Geometry: final body of the model. Coordinates: model frame, mm. A direction names the side the tool comes from. Round coordinates to 2 decimals unless told otherwise and drop trailing zeros. Loops run counter-clockwise (first coordinate to the right, second up) from the corner with the lowest first, then second, coordinate; pieces in that order, holes last. Notation, with made-up numbers: (50, 67.25) -> (71, 67.25) arc R30 cw to (71, 104.25) -> close; hole circle Ø4 at (72, -36.5). An arc over 180 degrees is marked (long way). Answer in a Markdown table with one row per item.
```python
from build123d import *

# Parameters (mm, degrees)
F0_W     = 2
F0_H     = 2.4
F1_DEPTH = 10
F2_DEPTH = 10


with BuildPart() as f1:
    # F0 (on Top) → F1 (new body)
    with BuildSketch(Plane.XY):
        with Locations((-8.5, 4.8)):
            Rectangle(F0_W, F0_H)
        Polygon((-11.5, 0), (-9.5, 0), (-9.5, 3.6), (-9.5, 6), (-11.5, 6), align=None)
        Polygon((9.5, 0), (0, 0), (0, -1.5), (11.5, -1.5), (11.5, 0), align=None)
        with Locations((8.5, 4.8)):
            Rectangle(F0_W, F0_H)
        Polygon((0, -1.5), (0, 0), (-9.5, 0), (-11.5, 0), (-11.5, -1.5), align=None)
        Polygon((9.5, 3.6), (9.5, 0), (11.5, 0), (11.5, 6), (9.5, 6), align=None)
    extrude(amount=F1_DEPTH)

    # F0 (on Top) → F2 (join)
    with BuildSketch(Plane.XY):
        Polygon((-11.5, -1.5), (-11.5, 0), (-11.5, 6), (-19, 6), (-16, -1.5), align=None)
        with BuildLine():
            Line((-31, 6), (-28, 6))
            Line((-28, 6), (-28, 28.5))
            Line((-28, 28.5), (-28, 53.5))
            ThreePointArc((-28, 53.5), (-33, 58.5), (-38, 53.5))
            Line((-38, 53.5), (-38, 23.5))
            Line((-38, 23.5), (-31, 6))
        make_face()
        Polygon((11.5, 0), (11.5, -1.5), (16, -1.5), (19, 6), (11.5, 6), align=None)
        with BuildLine():
            Line((28, 6), (31, 6))
            Line((31, 6), (38, 23.5))
            Line((38, 23.5), (38, 53.5))
            ThreePointArc((38, 53.5), (33, 58.5), (28, 53.5))
            Line((28, 53.5), (28, 28.5))
            Line((28, 28.5), (28, 6))
        make_face()
        Polygon((-28, 6), (-19, 6), (-28, 28.5), align=None)
        Polygon((-28, -1.5), (-16, -1.5), (-19, 6), (-28, 6), (-31, 6), align=None)
        Polygon((19, 6), (16, -1.5), (28, -1.5), (31, 6), (28, 6), align=None)
        Polygon((28, 28.5), (19, 6), (28, 6), align=None)
        Polygon((11.5, -1.5), (0, -1.5), (-11.5, -1.5), (-16, -1.5), (-28, -1.5), (-26.5144372946, -5.2139067635), (26.5144372946, -5.2139067635), (28, -1.5), (16, -1.5), align=None)
    extrude(amount=F2_DEPTH)


solid = f1.part
```
Item 1: Section query C-C, the plane x = 22.5. Output: boundary loops of the cut face in (y, z), and give its area (3 significant figures).
Ans:
| item | result |
|---|---|
| outline | (-5.21, 0) -> (14.75, 0) -> (14.75, 10) -> (-5.21, 10) -> close |
| area | 200 mm2 |
Item 2: Set-up query: faces 4 (the flat face through (-23.437, 17.092, 4.93)), 5 (the flat face through (0, -5.214, 5)), 6 (the flat face through (0, 0, 5)). Return all of +Z, -Z, +X, -X, +Y, -Y with unobstructed straight access to the full face (end or side cutting, diameter ignored); none if empty.
Ans:
| item | result |
|---|---|
| face 4 | +Z, -Z, +Y |
| face 5 | +Z, -Z, +X, -X, -Y |
| face 6 | +Z, -Z |
Item 3: Section query D-D, the plane x = -33. Output: boundary loops of the cut face in (y, z).
Ans:
| item | result |
|---|---|
| outline | (11, 0) -> (58.5, 0) -> (58.5, 10) -> (11, 10) -> close |
Item 4: Section query A-A, the plane y = 19.5. Output: boundary loops of the cut face in (x, z), and give its area (3 significant figures).
Ans:
| item | result |
|---|---|
| outline | (-36.4, 0) -> (-24.4, 0) -> (-24.4, 10) -> (-36.4, 10) -> close; (24.4, 0) -> (36.4, 0) -> (36.4, 10) -> (24.4, 10) -> close |
| area | 240 mm2 |
Item 5: Ray query, L1, parallel to X at y = 40.5, z = 2.5; L2, parallel to X at y = 2, z = 9.75; L3, parallel to Y at x = 5.5, z = 9. Return the intervals inside material, ascending.
Ans:
| item | result |
|---|---|
| L1 | -38 to -28, 28 to 38 |
| L2 | -29.4 to -9.5, 9.5 to 29.4 |
| L3 | -5.21 to 0 |
Item 6: First-contact query: P1, Ø3, axis at y = 1, z = 6.5, coming from the +X side; P2, Ø5, axis at x = -13, z = 5, coming from the +Y side; P3, Ø3, axis at x = -3, z = 4, coming from the +Y side. Flat tips, straight axial feed; report the tip coordinate or a pass-through.
Ans:
| item | result |
|---|---|
| P1 | x = 29.6 |
| P2 | y = 6 |
| P3 | y = 0 |
Item 7: Section query B-B, the plane z = 9. Output: boundary loops of the cut face in (x, y).
Ans:
| item | result |
|---|---|
| outline | (-38, 23.5) -> (-26.51, -5.21) -> (26.51, -5.21) -> (38, 23.5) -> (38, 53.5) arc R5 ccw to (28, 53.5) -> (28, 28.5) -> (19, 6) -> (7.5, 6) -> (7.5, 3.6) -> (9.5, 3.6) -> (9.5, 0) -> (-9.5, 0) -> (-9.5, 3.6) -> (-7.5, 3.6) -> (-7.5, 6) -> (-19, 6) -> (-28, 28.5) -> (-28, 53.5) arc R5 ccw to (-38, 53.5) -> close |
Item 8: Mould query, pull axis X, two halves, no side actions, for faces 1 (the flat face through (9.5, 2, 5)), 2 (the flat face through (7.91, 5.85, 0)), 3 (the flat face through (38, 38, 5)). Classes: released by +X, released by -X, zero draft, split by the parting line, or undercut.
Ans:
| item | result |
|---|---|
| face 1 | undercut |
| face 2 | zero draft |
| face 3 | released by +X |
